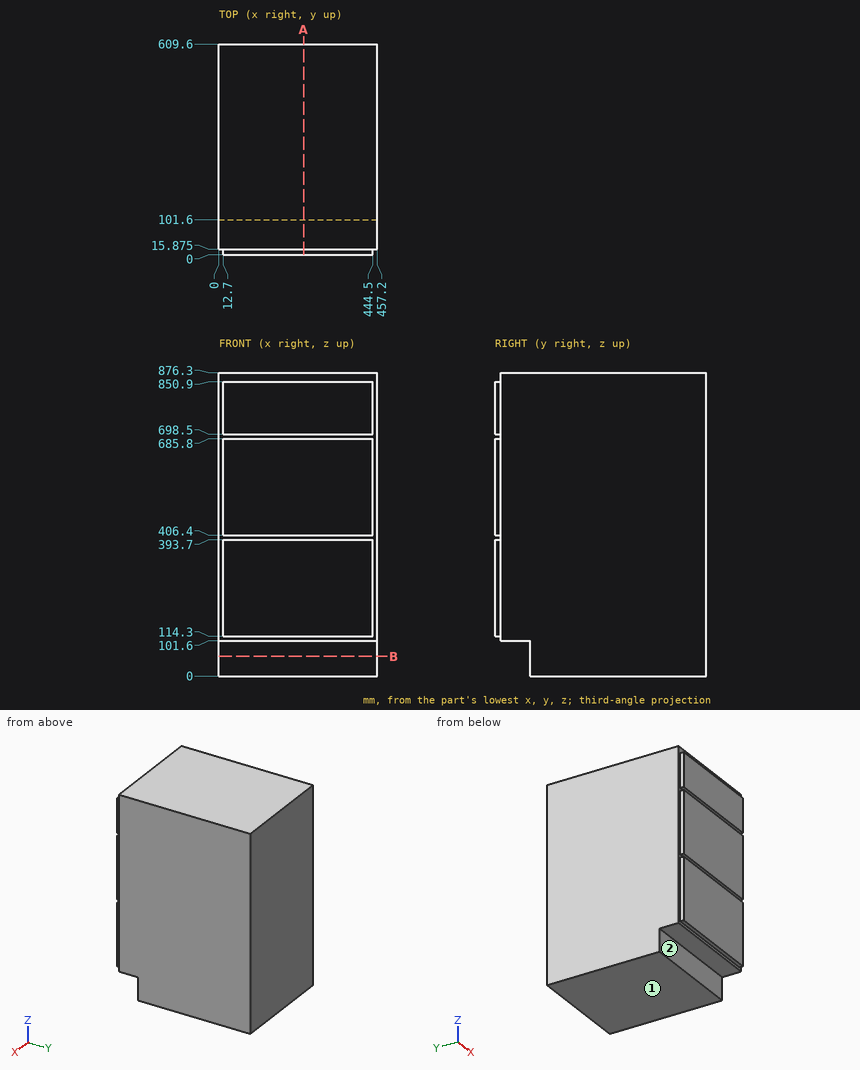
For this review, use the dimensioned drawing (mm, ordinates from the lowest corner) and the shaded views. A direction names the side the tool comes from. Round coordinates to 2 decimals unless told otherwise and drop trailing zeros. Order: outer loops, then holes, each group sorted by start corner. A loop starts at its lowest first (then second) coordinate and runs counter-clockwise, first axis right, second up.
1) Machinability: for the marked faces 1 and 2, which of the approach directions +Z, -Z, +X, -X, +Y, -Y give a long, thin tool a straight path to every point of the face, cutting with its end or side? Answer none if there is none.
The answers:
face 1: -Z, +X, -X, +Y, -Y
face 2: -Z, +X, -X, -Y
2) Clearance check with flat-ended pins moving along their axes: pin 1 Ø12.5 at (y, z) = (4.5, 487.5) entering from -X; pin 2 Ø4 at (x, y) = (303.5, 344) entering from -Z; pin 3 Ø5 at (x, y) = (276.5, 9) entering from -Z; pin 4 Ø17.5 at (x, y) = (171.5, 11) entering from -Z. State where each tip first meets the part, or that it passes through.
The answers:
pin 1: stops at x = 12.7
pin 2: stops at z = 0
pin 3: stops at z = 114.3
pin 4: stops at z = 101.6
3) Consider section A-A (x = 245). State the section outline as (y, z) points (3 decimals).
The answers:
outline: (0, 114.3) - (15.875, 114.3) - (15.875, 101.6) - (101.6, 101.6) - (101.6, 0) - (609.6, 0) - (609.6, 876.3) - (15.875, 876.3) - (15.875, 850.9) - (0, 850.9) - (0, 698.5) - (15.875, 698.5) - (15.875, 685.8) - (0, 685.8) - (0, 406.4) - (15.875, 406.4) - (15.875, 393.7) - (0, 393.7) - close
4) For L1, parallel to Y at x = 203, z = 63.5; L2, parallel to Z at x = 345.5, y = 59; L3, parallel to Y at x = 292, z = 396 (3 decimals), list the stretches that pass through material, from the lowest coordinate up.
The answers:
L1: y = 101.6 to 609.6
L2: z = 101.6 to 876.3
L3: y = 15.875 to 609.6
5) Consider section B-B (z = 57). State the section outline as (x, y) points.
The answers:
outline: (0, 101.6) - (457.2, 101.6) - (457.2, 609.6) - (0, 609.6) - close
